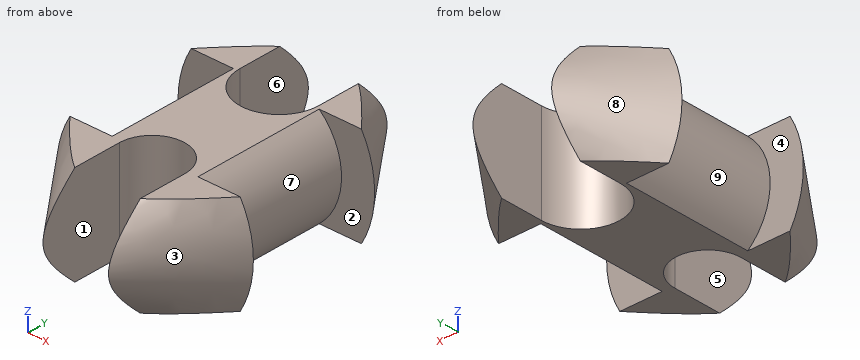
from build123d import *

# Parameters (mm, degrees)
ESBO_O2_OUTSIDE_W          = 45.13
ESBO_O2_OUTSIDE_H          = 45.13
ESBO_O2_OUTSIDE_W_2        = 30
ESBO_O2_OUTSIDE_H_2        = 15
CORTE_EXTRUS_O1_DEPTH      = 26.05
CORTE_EXTRUS_O1_DEPTH_BACK = 26.05
CORTE_EXTRUS_O2_DEPTH      = 16


with BuildPart() as part:
    # Esboço1 one side → Revolução1 (revolve)
    with BuildSketch(Plane.XY):
        with BuildLine():
            ThreePointArc((4, 24.506832295), (2.018355219, 24.913587797), (0, 25.05))
            Line((0, 25.05), (0, -25.05))
            ThreePointArc((0, -25.05), (2.018355219, -24.913587797), (4, -24.506832295))
            Line((4, -24.506832295), (15, -10.05))
            Line((15, -10.05), (9.95, -10.05))
            Line((9.95, -10.05), (9.95, 10.05))
            Line((9.95, 10.05), (15, 10.05))
            Line((15, 10.05), (4, 24.506832295))
        make_face()
    revolve(axis=Axis((0, -25.05, 0), (0, 1, 0)))

    # Esboço2 outside → Corte-extrusão1 (cut, two sides)
    with BuildSketch(Plane(origin=(0, 0, 0), x_dir=(1, 0, 0), z_dir=(0, 1, 0))) as corte_extrus_o1_sk:
        Rectangle(ESBO_O2_OUTSIDE_W, ESBO_O2_OUTSIDE_H)
        Rectangle(ESBO_O2_OUTSIDE_W_2, ESBO_O2_OUTSIDE_H_2, mode=Mode.SUBTRACT)
    extrude(amount=CORTE_EXTRUS_O1_DEPTH, mode=Mode.SUBTRACT)
    extrude(corte_extrus_o1_sk.sketch, amount=-CORTE_EXTRUS_O1_DEPTH_BACK, mode=Mode.SUBTRACT)

    # Esboço3 → Corte-extrusão2 (cut, through all)
    with BuildSketch(Plane(origin=(0, 0, -7.5), x_dir=(-1, 0, 0), z_dir=(0, 0, -1))):
        with BuildLine():
            Line((6, 25.05), (6, 10.55))
            ThreePointArc((6, 10.55), (0, 4.55), (-6, 10.55))
            Line((-6, 10.55), (-6, 25.05))
            ThreePointArc((-6, 25.05), (0, 31.05), (6, 25.05))
        make_face()
        with BuildLine():
            Line((-5, -25.05), (-5, -10.55))
            ThreePointArc((-5, -10.55), (0, -5.55), (5, -10.55))
            Line((5, -10.55), (5, -25.05))
            ThreePointArc((5, -25.05), (0, -30.05), (-5, -25.05))
        make_face()
    extrude(amount=-CORTE_EXTRUS_O2_DEPTH, mode=Mode.SUBTRACT)


solid = part.part
Design review of the part built by this model. Coordinates are the model's own, in mm. Face numbers are marked on the shaded views. A direction names the side the tool comes from. Round coordinates to 2 decimals unless told otherwise and drop trailing zeros. Write each loop counter-clockwise with the first axis right and the second up, starting at its lowest first coordinate (ties: lowest second). Pieces come first, ordered by that corner, then holes. Notation, with made-up numbers: (-12, 40) - (41, 40) arc R24 cw to (41, 52) - close; hole circle Ø5 at (81.25, 73.25). An arc over 180 degrees is marked (long way). Return JSON: item names as keys, results as strings. Group by question number.
Item 1: We need section A-A on y = 8. Write out the cut boundary in (x, z).
Item 2: For probe 1 along X at (y, z) = (-5.5, 0.25); probe 2 along X at (y, z) = (-13, -5.5); probe 3 along Y at (x, z) = (13, -4.25), list the stretches that pass through material, from the lowest coordinate up. Write a range as [from, to].
Item 3: Machinability: for the marked faces 5, 6, 7, 8 and 9, which of the approach directions +Z, -Z, +X, -X, +Y, -Y give a long, thin tool a straight path to every point of the face, cutting with its end or side? Answer none if there is none.
Item 4: We need section C-C on y = -9.5. Write out the cut boundary in (x, z), and give its area (3 significant figures).
Item 5: We need section B-B on x = 0. Write out the cut boundary in (y, z), and give its area (4 significant figures).
Item 6: The part is to be moulded in two halves that separate along Y. For the marked faces 1, 2, 3 and 4, say which applies: pulls with the +Y half, pulls with the -Y half, needs draft (parallel to the pull), parting line crosses it, or undercut.
Item 7: Insertion check: P1, Ø5.5, axis at y = 15, z = 2, coming from the -X side; P2, Ø8, axis at y = 1, z = 1, coming from the +X side; P3, Ø3, axis at x = 12, z = 3, coming from the -Y side. Each pin has a flat end and moves straight along its axis. Give the tip position at first contact, or say it passes through.
Model answer:
{
 "1": {"outline": "(-6.54, -7.5) - (-5.43, -7.5) - (-5.43, 7.5) - (-6.54, 7.5) arc R9.95 ccw to start; (5.43, -7.5) - (6.54, -7.5) arc R9.95 ccw to (6.54, 7.5) - (5.43, 7.5) - close"},
 "2": {"probe 1": "x = [-9.95, 9.95]", "probe 2": "x = [-11.51, -5], [5, 11.51]", "probe 3": "y = [-11.79, -10.05], [10.05, 11.79]"},
 "3": {"face 5": "+Z, -Z, -Y", "face 6": "+Z, -Z, +Y", "face 7": "+X", "face 8": "-X, +Y", "face 9": "-X"},
 "4": {"outline": "(-6.54, -7.5) - (-4.89, -7.5) - (-4.89, 7.5) - (-6.54, 7.5) arc R9.95 ccw to start; (4.89, -7.5) - (6.54, -7.5) arc R9.95 ccw to (6.54, 7.5) - (4.89, 7.5) - close", "area": "120 mm²"},
 "5": {"outline": "(-5.55, -7.5) - (4.55, -7.5) - (4.55, 7.5) - (-5.55, 7.5) - close", "area": "151.5 mm²"},
 "6": {"face 1": "needs draft", "face 2": "undercut", "face 3": "pulls with the -Y half", "face 4": "undercut"},
 "7": {"P1": "stops at x = -13.21", "P2": "stops at x = 9.95", "P3": "stops at y = -15.48"}
}
